```python
from build123d import *

# Parameters (mm, degrees)
SKETCH3_R          = 14.224
BASE_EXTRUDE_DEPTH = 15.875
SKETCH4_W          = 2.286
SKETCH4_H          = 2.286
SKETCH5_R          = 3.175
CUT_EXTRUDE1_DEPTH = 26.625377597
CHAMFER1_SIZE      = 0.762


with BuildPart() as part:
    # Sketch3 → Base-Extrude (new body)
    with BuildSketch(Plane(origin=(0, 0, 0), x_dir=(0, 0, -1), z_dir=(1, 0, 0))):
        Circle(SKETCH3_R)
    extrude(amount=BASE_EXTRUDE_DEPTH)

    # Sketch4 → Cut-Revolve1 (revolve, cut)
    with BuildSketch(Plane.XY, mode=Mode.PRIVATE) as cut_revolve1_sk:
        with Locations((4.191, 13.081)):
            Rectangle(SKETCH4_W, SKETCH4_H)
        with Locations((11.684, 13.081)):
            Rectangle(SKETCH4_W, SKETCH4_H)
    revolve(cut_revolve1_sk.sketch.rotate(Axis((0, 0, 0), (1, 0, 0)), 90), axis=Axis((0, 0, 0), (1, 0, 0)), mode=Mode.SUBTRACT)

    # Sketch5 → Cut-Extrude1 (cut, through all)
    with BuildSketch(Plane.ZY):
        Circle(SKETCH5_R)
    extrude(amount=-CUT_EXTRUDE1_DEPTH, mode=Mode.SUBTRACT)

    # Chamfer1
    chamfer1_edges = [part.edges().sort_by_distance(p)[0] for p in [
        (0, 0, 14.224),
        (15.875, 0, 14.224),
    ]]
    chamfer(chamfer1_edges, length=CHAMFER1_SIZE)


solid = part.part
```
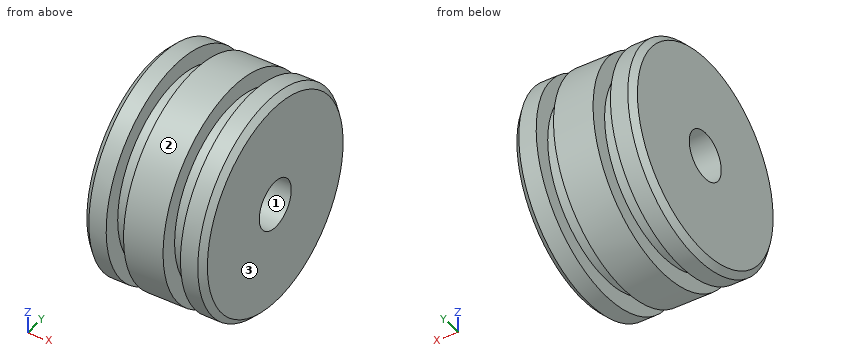
Source: CAD feature listing. Evaluate the final solid. Frame: model axes, mm. Face numbers are marked on the shaded views. Round coordinates to 2 decimals unless told otherwise and drop trailing zeros. Loops run counter-clockwise (first coordinate to the right, second up) from the corner with the lowest first, then second, coordinate; pieces in that order, holes last.
1. Section query A-A on y = 0. Output: boundary loops of the cut face in (x, z) (3 decimals), and give its area (3 significant figures).
2. Section query C-C on x = 11.75. Output: boundary loops of the cut face in (y, z) (3 decimals).
3. Mould query, pull axis Z, two halves, no side actions, for the marked faces 1, 2 and 3. Classes: released by +Z, released by -Z, zero draft, split by the parting line, or undercut.
4. Contact query for flat-ended pins moving along their axis: pin 1 (3 mm diameter, centred on x = 4, z = 10, fed in from -Y); pin 2 (3 mm diameter, centred on x = 4.5, z = -2.5, fed in from -Y); pin 3 (1 mm diameter, centred on x = 13.5, z = -2.5, fed in from +Y). Output: stop coordinate, or through.
5. Section query D-D on x = 13.75. Output: boundary loops of the cut face in (y, z) (3 decimals).
6. Ray query, L1, parallel to X at y = -5.5, z = 10.75 (3 decimals); L2, parallel to Y at x = 10, z = 0 (3 decimals); L3, parallel to X at y = -11.25, z = 8. Return the intervals inside material, ascending.
Answers below:
1. outline: (0, -13.462) - (0.762, -14.224) - (3.048, -14.224) - (3.048, -11.938) - (5.334, -11.938) - (5.334, -14.224) - (10.541, -14.224) - (10.541, -11.938) - (12.827, -11.938) - (12.827, -14.224) - (15.113, -14.224) - (15.875, -13.462) - (15.875, -3.175) - (0, -3.175) - close; (0, 3.175) - (15.875, 3.175) - (15.875, 13.462) - (15.113, 14.224) - (12.827, 14.224) - (12.827, 11.938) - (10.541, 11.938) - (10.541, 14.224) - (5.334, 14.224) - (5.334, 11.938) - (3.048, 11.938) - (3.048, 14.224) - (0.762, 14.224) - (0, 13.462) - close
1. area: 329 mm2
2. outline: circle Ø23.876 at (0, 0); hole circle Ø6.35 at (0, 0)
3. face 1: undercut
3. face 2: split by the parting line
3. face 3: zero draft
4. pin 1: stops at y = -11.14
4. pin 2: stops at y = -14.17
4. pin 3: stops at y = 14.08
5. outline: circle Ø28.448 at (0, 0); hole circle Ø6.35 at (0, 0)
6. L1: x = 0 to 3.048, 5.334 to 10.541, 12.827 to 15.875
6. L2: y = -14.224 to -3.175, 3.175 to 14.224
6. L3: x = 0.34 to 3.05, 5.33 to 10.54, 12.83 to 15.53
